Source: CAD feature listing. Evaluate the final solid. Frame: model axes, mm. Face numbers are marked on the shaded views. A direction names the side the tool comes from. Coordinates: 2 decimals unless noted, no trailing zeros. Write each loop counter-clockwise with the first axis right and the second up, starting at its lowest first coordinate (ties: lowest second). Pieces come first, ordered by that corner, then holes. Notation, with made-up numbers: (82.5, -10.5) -> (141.5, -10.5) arc R15 ccw to (141.5, -3.5) -> close; hole circle Ø8 at (45, 22.5). An arc over 180 degrees is marked (long way). One line per item, written item: value. Start each with the question number.
1. Mould query, pull axis X, two halves, no side actions, for the marked faces 1, 2, 3 and 4. Classes: released by +X, released by -X, zero draft, split by the parting line, or undercut.
2. Access query for the marked faces 5, 6 and 7. Directions: +Z, -Z, +X, -X, +Y, -Y. A direction counts if a zero-diameter tool reaches every point of the face in a straight line with its end or side. Return the directions, or none.
3. Section query B-B, the plane x = -49. Output: boundary loops of the cut face in (y, z), and give its area (3 significant figures).
4. First-contact query: P1, Ø3.5, axis at y = -8.5, z = 1, coming from the -X side; P2, Ø6, axis at x = -9.5, y = 85, coming from the +Z side; P3, Ø4, axis at x = 32.5, z = 20, coming from the +Y side; P4, Ø3.5, axis at x = 62.5, y = 94.55, coming from the +Z side. Flat tips, straight axial feed; report the tip coordinate or a pass-through.
5. Section query A-A, the plane y = -21.5. Output: boundary loops of the cut face in (x, z).
6. Line query: line 1 (Y direction, x = 62.5, z = 8.25); line 2 (Y direction, x = 62.5, z = 3); line 3 (Y direction, x = -28.5, z = 8). Output: solid intervals per line, ascending.
7. Section query C-C, the plane z = 40. Output: boundary loops of the cut face in (x, y).
8. Section query D-D, the plane x = -70. Output: boundary loops of the cut face in (y, z).
from build123d import *

# Parameters (mm, degrees)
SKIZZE1_R                       = 2.3
SKIZZE1_R_2                     = 5
SKIZZE1_R_3                     = 2.75
SKIZZE1_W                       = 43.1
SKIZZE1_H                       = 63
AUFSATZ_LINEAR_AUSTRAGEN1_DEPTH = 10
AUFSATZ_LINEAR_AUSTRAGEN3_DEPTH = 10
SKIZZE4_W                       = 110
SKIZZE4_H                       = 15.089693508
AUFSATZ_LINEAR_AUSTRAGEN4_DEPTH = 100
VERRUNDUNG5_R                   = 10
SKIZZE11_R                      = 4.5
SCHNITT_LINEAR_AUSTRAGEN1_DEPTH = 3
SCHNITT_LINEAR_AUSTRAGEN2_DEPTH = 3
AUFSATZ_LINEAR_AUSTRAGEN7_DEPTH = 10
AUFSATZ_LINEAR_AUSTRAGEN8_DEPTH = 10


with BuildPart() as part:
    # Skizze1 → Aufsatz-Linear austragen1 (new body)
    with BuildSketch(Plane.XY):
        with BuildLine():
            Line((90, 107.054645521), (-90, 107.054645521))
            ThreePointArc((-90, 107.054645521), (-97.071067812, 104.125713333), (-100, 97.054645521))
            Line((-100, 97.054645521), (-100, 77.054645521))
            ThreePointArc((-100, 77.054645521), (-97.071067812, 69.983577709), (-90, 67.054645521))
            Line((-90, 67.054645521), (-70, 67.054645521))
            ThreePointArc((-70, 67.054645521), (-59.393398282, 62.661247239), (-55, 52.054645521))
            Line((-55, 52.054645521), (-55, -82.945354479))
            Line((-55, -82.945354479), (55, -82.945354479))
            Line((55, -82.945354479), (55, 52.054645521))
            ThreePointArc((55, 52.054645521), (59.393398282, 62.661247239), (70, 67.054645521))
            Line((70, 67.054645521), (90, 67.054645521))
            ThreePointArc((90, 67.054645521), (97.071067812, 69.983577709), (100, 77.054645521))
            Line((100, 77.054645521), (100, 97.054645521))
            ThreePointArc((100, 97.054645521), (97.071067812, 104.125713333), (90, 107.054645521))
        make_face()
        with Locations((-28.5, 13.704645521)):
            Circle(SKIZZE1_R, mode=Mode.SUBTRACT)
        with Locations((-28.5, -9.295354479)):
            Circle(SKIZZE1_R, mode=Mode.SUBTRACT)
        with Locations(Location((28.5, -9.295354479, 0), (0, 0, 180))):
            Circle(SKIZZE1_R, mode=Mode.SUBTRACT)
        with Locations(Location((28.5, 13.704645521, 0), (0, 0, 180))):
            Circle(SKIZZE1_R, mode=Mode.SUBTRACT)
        with Locations((-70, 87.054645521)):
            Circle(SKIZZE1_R_2, mode=Mode.SUBTRACT)
        with Locations((-62.5, 94.554645521)):
            Circle(SKIZZE1_R_3, mode=Mode.SUBTRACT)
        with Locations((-77.5, 79.554645521)):
            Circle(SKIZZE1_R_3, mode=Mode.SUBTRACT)
        with Locations(Location((77.5, 79.554645521, 0), (0, 0, 180))):
            Circle(SKIZZE1_R_3, mode=Mode.SUBTRACT)
        with Locations(Location((62.5, 94.554645521, 0), (0, 0, 180))):
            Circle(SKIZZE1_R_3, mode=Mode.SUBTRACT)
        with Locations(Location((70, 87.054645521, 0), (0, 0, 180))):
            Circle(SKIZZE1_R_2, mode=Mode.SUBTRACT)
        with Locations((0, 2.204645521)):
            Rectangle(SKIZZE1_W, SKIZZE1_H, mode=Mode.SUBTRACT)
    extrude(amount=AUFSATZ_LINEAR_AUSTRAGEN1_DEPTH)

    # Skizze3 → Aufsatz-Linear austragen3 (add)
    with BuildSketch(Plane.XY.offset(10)):
        with BuildLine():
            Line((-72.845922337, 57.814606503), (-56.774282723, 37.352261221))
            add(Edge.make_bspline(
                [(-55, 18.961003518), (-46.636539725, 27.963101216), (-56.774282723, 37.352261221)],
                knots=[0, 0, 0, 1, 1, 1], degree=2))
            Line((-55, 18.961003518), (-43.333440031, 21.200490786))
            Line((-43.333440031, 21.200490786), (-45.498025685, 67.054645521))
            Line((-45.498025685, 67.054645521), (-90, 67.054645521))
            add(Edge.make_bspline(
                [(-90, 67.054645521), (-79.938268155, 65.656359823), (-72.845922337, 57.814606503)],
                knots=[0, 0, 0, 1, 1, 1], degree=2))
        make_face()
    extrude(amount=-AUFSATZ_LINEAR_AUSTRAGEN3_DEPTH)

    # Skizze4 → Aufsatz-Linear austragen4 (add)
    with BuildSketch(Plane.XY.offset(10)):
        with Locations((0, -75.400507725)):
            Rectangle(SKIZZE4_W, SKIZZE4_H)
    extrude(amount=AUFSATZ_LINEAR_AUSTRAGEN4_DEPTH)

    # Verrundung5
    # the kernel refuses this fillet: 10 mm, written as the material it adds along each edge
    with BuildSketch(Plane(origin=(-55, 35.554962551, 0), x_dir=(-0.702535464065595, 0.7116487347913572, 0), z_dir=(0, 0, 1))) as verrundung5_piece_1:
        with BuildLine():
            CenterArc((4.257528526, 9.848869082), VERRUNDUNG5_R, 225.36921974, 34.65693161)
            Line((-2.767826115, 2.732381734), (-2.908333207, 2.590051987))
            Line((-2.908333207, 2.590051987), (-0.140507093, -0.142329747))
            Line((-0.140507093, -0.142329747), (-0.009856246, -0.199756988))
            ThreePointArc((-0.009856246, -0.199756988), (1.263031351, -0.229630028), (2.490902127, -0.196977382))
            Line((2.490902127, -0.196977382), (2.52554186, 0))
        make_face()
    extrude(amount=10)

    # Skizze11 → Schnitt-Linear austragen1 (cut)
    with BuildSketch(Plane.XY.offset(10)):
        with Locations((62.5, 94.554645521)):
            Circle(SKIZZE11_R)
        with Locations((77.5, 79.554645521)):
            Circle(SKIZZE11_R)
        with Locations((-62.5, 94.554645521)):
            Circle(SKIZZE11_R)
        with Locations((-77.5, 79.554645521)):
            Circle(SKIZZE11_R)
    extrude(amount=-SCHNITT_LINEAR_AUSTRAGEN1_DEPTH, mode=Mode.SUBTRACT)

    # Skizze12 → Schnitt-Linear austragen2 (cut)
    with BuildSketch(Plane(origin=(0, 0, 0), x_dir=(-1, 0, 0), z_dir=(0, 0, -1))):
        Polygon((28.5, 17.747145521), (24.825, 15.787145521), (24.825, 11.622145521), (28.5, 9.662145521), (32.175, 11.622145521), (32.175, 15.787145521), align=None)
        Polygon((28.5, -5.252854479), (24.825, -7.212854479), (24.825, -11.377854479), (28.5, -13.337854479), (32.175, -11.377854479), (32.175, -7.212854479), align=None)
        Polygon((-28.5, -5.252854479), (-32.175, -7.212854479), (-32.175, -11.377854479), (-28.5, -13.337854479), (-24.825, -11.377854479), (-24.825, -7.212854479), align=None)
        Polygon((-28.5, 17.747145521), (-32.175, 15.787145521), (-32.175, 11.622145521), (-28.5, 9.662145521), (-24.825, 11.622145521), (-24.825, 15.787145521), align=None)
    extrude(amount=-SCHNITT_LINEAR_AUSTRAGEN2_DEPTH, mode=Mode.SUBTRACT)

    # Skizze15 → Aufsatz-Linear austragen7 (add)
    with BuildSketch(Plane.ZY.offset(55)):
        Polygon((10, 2.144339029), (80, -67.855660971), (10, -67.855660971), align=None)
    extrude(amount=-AUFSATZ_LINEAR_AUSTRAGEN7_DEPTH)

    # Skizze16 → Aufsatz-Linear austragen8 (add)
    with BuildSketch(Plane(origin=(55, 0, 0), x_dir=(0, 0, -1), z_dir=(1, 0, 0))):
        Polygon((-10, 2.204645521), (-80, -67.855660971), (-10, -67.855660971), align=None)
    extrude(amount=-AUFSATZ_LINEAR_AUSTRAGEN8_DEPTH)


solid = part.part
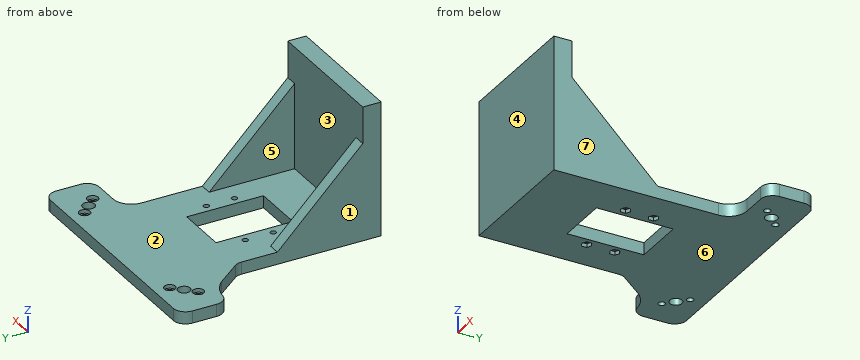
Computed values:
1. face 1: released by -X
1. face 2: undercut
1. face 3: undercut
1. face 4: zero draft
2. face 5: +Z, +Y
2. face 6: -Z, +X, -X, +Y, -Y
2. face 7: +Z, -Z, +X, -Y
3. outline: (-82.95, 0) -> (107.05, 0) -> (107.05, 10) -> (2.14, 10) -> (-67.86, 80) -> (-67.86, 110) -> (-82.95, 110) -> close
3. area: 5,860 mm²
4. P1: stops at x = -55
4. P2: stops at z = 10
4. P3: stops at y = -67.86
4. P4: passes through
5. outline: (-55, 0) -> (-21.55, 0) -> (-21.55, 10) -> (-45, 10) -> (-45, 33.64) -> (-55, 33.64) -> close; (21.55, 0) -> (55, 0) -> (55, 33.68) -> (45, 33.68) -> (45, 10) -> (21.55, 10) -> close
6. line 1: y = 65.05 to 90.05, 99.05 to 107.05
6. line 2: y = 65.05 to 91.8, 97.3 to 107.05
6. line 3: y = -82.95 to -11.6, -7 to 11.4, 16 to 107.05
7. outline: (-55, -82.95) -> (55, -82.95) -> (55, -27.82) -> (45, -27.82) -> (45, -67.86) -> (-45, -67.86) -> (-45, -27.86) -> (-55, -27.86) -> close
8. outline: (54.19, 0) -> (82.05, 0) -> (82.05, 10) -> (54.19, 10) -> close; (92.05, 0) -> (107.05, 0) -> (107.05, 10) -> (92.05, 10) -> close
